Work out the finished part from the listing and answer in its coordinate system (mm). A direction names the side the tool comes from. Coordinates: 2 decimals unless noted, no trailing zeros. Order: outer loops, then holes, each group sorted by start corner. A loop starts at its lowest first (then second) coordinate and runs counter-clockwise, first axis right, second up.
1. A tool of negligible diameter and unlimited length cuts with its end or side. For faces 4 (the conical face through (-23.319, 8.246, 4.858)), 5 (the flat face through (8, -1.75, 0)), from which of +Z, -Z, +X, -X, +Y, -Y can it reach the whole face along a straight path? Write none if from no direction.
2. Find the intervals of material crossed by probe 1 along X at (y, z) = (0, 0); probe 2 along Y at (x, z) = (-17.5, 2.75); probe 3 along Y at (x, z) = (9, -2.75), in increasing order.
3. Determine the mould class of faces 1 (the conical face through (-23.319, -8.246, -4.858)), 2 (the flat face through (0, 2, -5)), 3 (the conical face through (-19.849, -0.522, -2.656)) for opening direction X: +X half, -X half, draft (parallel to the pull), parting line (faces both ways), or undercut.
4. The part is cut by section B-B, the plane z = 4. Count the separate pieces of the cut face and the enclosed holes in it, then the cut area to 3 significant figures.
5. The part is cut by section A-A, the plane x = -17.5. Give the vertices of the cut face in (y, z).
6. Flat-ended cylindrical pins translate along their axes: pin 1 Ø7 at (x, y) = (-17.5, 0) entering from -Z; pin 2 Ø1.5 at (y, z) = (4, -1.5) entering from +X; pin 3 Ø4 at (x, z) = (17.5, 1.5) entering from +Y. Find the tip coordinate at first contact, or state that the pin passes through.
Autodesk Inventor part; units mm, degrees
ref_plane "YZ Plane" through (0, 0, 0) normal (1, 0, 0) x (0, 1, 0)
ref_plane "XZ Plane" through (0, 0, 0) normal (0, 1, 0) x (-1, 0, 0)
ref_plane "XY Plane" through (0, 0, 0) normal (0, 0, 1) x (1, 0, 0)
sketch "Sketch1" plane through (0, 0, 0) normal (1, 0, 0) x (0, 1, 0)
  line L0 (-10, 5) -> (10, 5)
  line L1 (10, 5) -> (10, -5)
  line L2 (10, -5) -> (-10, -5)
  line L3 (-10, -5) -> (-10, 5)
  line L4 (-10, 5) -> (10, -5) construction
  line L5 (10, 5) -> (-10, -5) construction
  point P0 (0, 0)
  dimension "Width" = 20
  dimension "Thickness" = 10
extrude "Extrusion1" add sketch "Sketch1" along normal mid plane 50
sketch "Sketch6" plane through (25, 10, -5) normal (0, 0, -1) x (-1, 0, 0)
  line L0 (50, 0) -> (50, -20)
  line L1 (50, 0) -> (0, 0)
  point P0 (25, -10)
  point P1 (42.5, -10)
  dimension "d40" = 7.5
  dimension "d56" = 10
hole "Hole5" at (-17.5, 0, -5) direction (0, 0, 1) diameter 4.5 depth 10.65 tip angle 118 countersink diameter 9.5 countersink angle 90
sketch "Sketch7" plane through (-25, -10, 5) normal (0, 0, 1) x (1, 0, 0)
  point P0 (25, 10)
fillet "Fillet1" radius 10 2 edges at (25, 10, 0) (25, -10, 0)
sketch "Sketch9" plane through (-25, -10, -5) normal (0, 0, -1) x (-1, 0, 0)
  line L0 (-25, 10) -> (-40, 10) construction
  line L1 (-25, 11.75) -> (-40, 11.75)
  line L2 (-40, 8.25) -> (-25, 8.25)
  arc A0 (-25, 8.25) -> (-25, 11.75) centre (-25, 10) ccw
  arc A1 (-40, 11.75) -> (-40, 8.25) centre (-40, 10) ccw
  line L3 (0, 20) -> (0, 0)
  line L4 (-40, 0) -> (0, 0)
  point P0 (-32.5, 10)
  dimension "d58" = 15
  dimension "d59" = 25
  dimension "d60" = 10
  dimension "d62" = 3.5
extrude "Extrusion2" cut sketch "Sketch9" against normal blind 10
fillet "Fillet2" radius 5 2 edges at (-25, 10, 0) (-25, -10, 0)
chamfer "Chamfer1" distance 0.5 angle 45 12 edges at (-2.4997, 10, -5) (22.0712, 7.0712, -5) (-2.4997, -10, -5) (-23.5355, -8.5355, -5) (-25, 0, -5) (-23.5355, 8.5355, -5) (-2.4997, 10, 5) (22.0712, 7.0712, 5) (-2.4997, -10, 5) (-23.5355, -8.5355, 5) (-25, 0, 5) (-23.5355, 8.5355, 5)
properties part number "Bell Support Beam" material "Brass, Soft Yellow"
Geometry says:
1. face 4: +Z, -X, +Y
1. face 5: +Z, -Z
2. probe 1: x = -25 to -19.75, -15.25 to -1.75, 16.75 to 25
2. probe 2: y = -10 to -2.25, 2.25 to 10
2. probe 3: y = -10 to -1.75, 1.75 to 10
3. face 1: -X half
3. face 2: draft
3. face 3: undercut
4. separate pieces: 1
4. enclosed holes: 2
4. area: 868 mm2
5. outline: (-10, -4.5) - (-9.5, -5) - (-4.75, -5) - (-2.25, -2.5) - (-2.25, 5) - (-9.5, 5) - (-10, 4.5) - close; (2.25, -2.5) - (4.75, -5) - (9.5, -5) - (10, -4.5) - (10, 4.5) - (9.5, 5) - (2.25, 5) - close
6. pin 1: stops at z = -3.75
6. pin 2: stops at x = 24.46
6. pin 3: stops at y = 9.99
